For this review, take the finished solid that the model builds, in its own axes (mm). A direction names the side the tool comes from. Give positions to 0.01 mm unless a question says otherwise; leave off trailing zeros. Order: outer loops, then holes, each group sorted by start corner. A loop starts at its lowest first (then second) coordinate and runs counter-clockwise, first axis right, second up. Notation, with made-up numbers: (6, 30.25) -> (33, 30.25) arc R20 ccw to (33, 34.25) -> close; hole circle Ø5 at (34, -9). An arc over 180 degrees is marked (long way). Return JSON: item names as keys, results as strings. Group by question number.
1) Add section D-D (y = 0.25). Give the boundary of the cut face in (x, z) (3 decimals).
2) Insertion check: P1, Ø0.9, axis at y = 1.5, z = 6.5, coming from the -X side (3 decimals); P2, Ø1.9, axis at y = 1.5, z = 6, coming from the +X side; P3, Ø0.5, axis at x = -4.5, z = 1.5, coming from the +Y side. Each pin has a flat end and moves straight along its axis. Give the tip position at first contact, or say it passes through.
3) The part is to be moulded in two halves that separate along Z. For faces 1 (the face through (-2.875, 1, 6)), 2 (the face through (4.574, 1.648, -3.215)), 3 (the face through (-1, 1, 8)), say which applies: released by +Z, released by -Z, zero draft, split by the parting line, or undercut.
4) Add section C-C (y = 2.2). Give the boundary of the cut face in (x, z) (3 decimals).
5) To check wall thickness, follow line 1 along Z through (x, y) = (-3.5, 2.95); line 2 along Z through (x, y) = (0, 2.05); line 3 along X through (y, z) = (1.05, 6) (3 decimals). State the ranges of each line that lie inside material, in increasing order.
6) Add section A-A (z = 6). Give the boundary of the cut face in (x, y) (3 decimals).
7) For faces 4 (the face through (4.924, 2.88, -3.565)), 5 (the face through (1.125, 1, 6)), 6 (the face through (-2.574, 1.268, 7.715)), 7 (the face through (4.94, 2.88, 3.55)), list the 3-axis set-ups (+Z, -Z, +X, -X, +Y, -Y) from which the entire face can be reached by the end or side of a thin tool; tool diameter is ignored.
8) Add section B-B (x = 3). Give the boundary of the cut face in (y, z), then the cut area to 4 significant figures.
from build123d import *

# Parameters (mm, degrees)
SKETCH5_W                 = 11.25
SKETCH5_H                 = 8.5
EXTRUDE4_DEPTH            = 2.5
SKETCH19_W                = 1.5
SKETCH19_H                = 8.5
EXTRUDE12_DEPTH           = 2
SKETCH21_W                = 9
SKETCH21_H                = 7
EXTRUDE13_DEPTH           = 8.48018215
SKETCH22_W                = 4
SKETCH22_H                = 2.5
EXTRUDE14_DEPTH           = 3.75
EXTRUDE15_DEPTH           = 0.75
F_0_80_TAPPED_HOLE1_D     = 1.19126
F_0_80_TAPPED_HOLE1_DEPTH = 79.01
F_0_80_TAPPED_HOLE1_TIP   = 0.357890611
FILLET4_R                 = 1
FILLET5_R                 = 1


with BuildPart() as part:
    # Sketch5 → Extrude4 (new body)
    with BuildSketch(Plane(origin=(0, 0, 0), x_dir=(1, 0, 0), z_dir=(0, 1, 0))):
        Rectangle(SKETCH5_W, SKETCH5_H)
    extrude(amount=EXTRUDE4_DEPTH)

    # Sketch19 → Extrude12 (cut)
    with BuildSketch(Plane(origin=(0, 2.5, 0), x_dir=(-1, 0, 0), z_dir=(0, 1, 0))):
        with Locations((4.875, 0)):
            Rectangle(SKETCH19_W, SKETCH19_H)
    extrude(amount=-EXTRUDE12_DEPTH, mode=Mode.SUBTRACT)

    # Sketch21 → Extrude13 (cut, through all)
    with BuildSketch(Plane(origin=(0, 2.5, 0), x_dir=(-1, 0, 0), z_dir=(0, 1, 0))):
        with Locations((-0.375, 0)):
            Rectangle(SKETCH21_W, SKETCH21_H)
    extrude(amount=-EXTRUDE13_DEPTH, mode=Mode.SUBTRACT)

    # Sketch22 → Extrude14 (add)
    with BuildSketch(Plane.XY.offset(4.25)):
        with Locations((-0.875, 1.25)):
            Rectangle(SKETCH22_W, SKETCH22_H)
    extrude(amount=EXTRUDE14_DEPTH)

    # Sketch24 → Extrude15 (add)
    with BuildSketch(Plane(origin=(0, 2.5, 0), x_dir=(1, 0, 0), z_dir=(0, 1, 0))):
        Polygon((-4.125, 3.85), (-4.125, 3.5), (4.875, 3.5), (4.875, -3.5), (-4.125, -3.5), (-4.125, -3.85), (5.225, -3.85), (5.225, 3.85), align=None)
    extrude(amount=EXTRUDE15_DEPTH)

    # #0-80 Tapped Hole1
    with Locations(Plane(origin=(-0.875, 2.5, 6), x_dir=(0, 0, 1), z_dir=(0, 1, 0))):
        with Locations((0, 0)):
            Hole(F_0_80_TAPPED_HOLE1_D / 2, depth=F_0_80_TAPPED_HOLE1_DEPTH)
            with Locations((0, 0, -(F_0_80_TAPPED_HOLE1_DEPTH + F_0_80_TAPPED_HOLE1_TIP / 2))):  # 118° drill point
                Cone(0, F_0_80_TAPPED_HOLE1_D / 2, F_0_80_TAPPED_HOLE1_TIP, mode=Mode.SUBTRACT)

    # Fillet4
    fillet4_edges = [part.edges().sort_by_distance(p)[0] for p in [
        (5.625, 1.25, -4.25),
        (5.225, 2.875, -3.85),
        (5.625, 1.25, 4.25),
        (5.225, 2.875, 3.85),
        (-2.875, 1.25, 8),
        (1.125, 1.25, 8),
        (1.125, 1.25, 4.25),
        (-2.875, 1.25, 4.25),
        (4.875, 1.625, 3.5),
        (4.875, 1.625, -3.5),
    ]]
    fillet(fillet4_edges, radius=FILLET4_R)

    # Fillet5
    # the kernel refuses this fillet: 1 mm, written as the material it takes off along each edge
    with BuildSketch(Plane(origin=(-5.625, 0.5, 6.415063509), x_dir=(0, -1, 0), z_dir=(0, 0, -1))) as fillet5_piece_1:
        with BuildLine():
            CenterArc((1, -0.866025404), FILLET5_R, 120, 60)
            Line((0, -0.866025404), (-0.02, -0.866025404))
            Line((-0.02, -0.866025404), (-0.02, 0))
            Line((-0.02, 0), (0, 0.02))
            ThreePointArc((0, 0.02), (0.25, 0.02), (0.49, 0.017320508))
            Line((0.49, 0.017320508), (0.5, 0))
        make_face()
    extrude(amount=12.830127019, mode=Mode.SUBTRACT)


solid = part.part
Evaluation:
{
 "1": {"outline": "(-5.42, -4.25) -> (4.625, -4.25) arc R1 ccw to (5.625, -3.25) -> (5.625, 3.25) arc R1 ccw to (4.625, 4.25) -> (2.125, 4.25) arc R1 cw to (1.125, 5.25) -> (1.125, 7) arc R1 ccw to (0.125, 8) -> (-1.875, 8) arc R1 ccw to (-2.875, 7) -> (-2.875, 5.25) arc R1 cw to (-3.875, 4.25) -> (-5.42, 4.25) -> close; hole (-4.125, -3.5) -> (3.875, -3.5) arc R1 ccw to (4.875, -2.5) -> (4.875, 2.5) arc R1 ccw to (3.875, 3.5) -> (-4.125, 3.5) -> close; hole circle Ø1.191 at (-0.875, 6)"},
 "2": {"P1": "x = -2.875", "P2": "x = 1.15", "P3": "y = 0.5"},
 "3": {"face 1": "zero draft", "face 2": "undercut", "face 3": "released by +Z"},
 "4": {"outline": "(-4.125, -4.25) -> (4.625, -4.25) arc R1 ccw to (5.625, -3.25) -> (5.625, 3.25) arc R1 ccw to (4.625, 4.25) -> (2.125, 4.25) arc R1 cw to (1.125, 5.25) -> (1.125, 7) arc R1 ccw to (0.125, 8) -> (-1.875, 8) arc R1 ccw to (-2.875, 7) -> (-2.875, 5.25) arc R1 cw to (-3.875, 4.25) -> (-4.125, 4.25) -> (-4.125, 3.5) -> (3.875, 3.5) arc R1 cw to (4.875, 2.5) -> (4.875, -2.5) arc R1 cw to (3.875, -3.5) -> (-4.125, -3.5) -> close; hole circle Ø1.191 at (-0.875, 6)"},
 "5": {"line 1": "-3.85 to -3.5, 3.5 to 3.85", "line 2": "-4.25 to -3.5, 3.5 to 8", "line 3": "-2.875 to -1.471, -0.279 to 1.125"},
 "6": {"outline": "(-2.875, 0) -> (-1.471, 0) -> (-1.471, 2.5) -> (-2.875, 2.5) -> close; (-0.279, 0) -> (1.125, 0) -> (1.125, 2.5) -> (-0.279, 2.5) -> close"},
 "7": {"face 4": "-Z, +X, +Y", "face 5": "+Z, +X, +Y, -Y", "face 6": "+Z, -X, +Y, -Y", "face 7": "+Z, +X, +Y"},
 "8": {"outline": "(0, -4.25) -> (2.5, -4.25) -> (2.5, -3.85) -> (3.25, -3.85) -> (3.25, -3.5) -> (0, -3.5) -> close; (0, 3.5) -> (3.25, 3.5) -> (3.25, 3.85) -> (2.5, 3.85) -> (2.5, 4.25) -> (0, 4.25) -> close", "area": "4.275 mm^2"}
}
